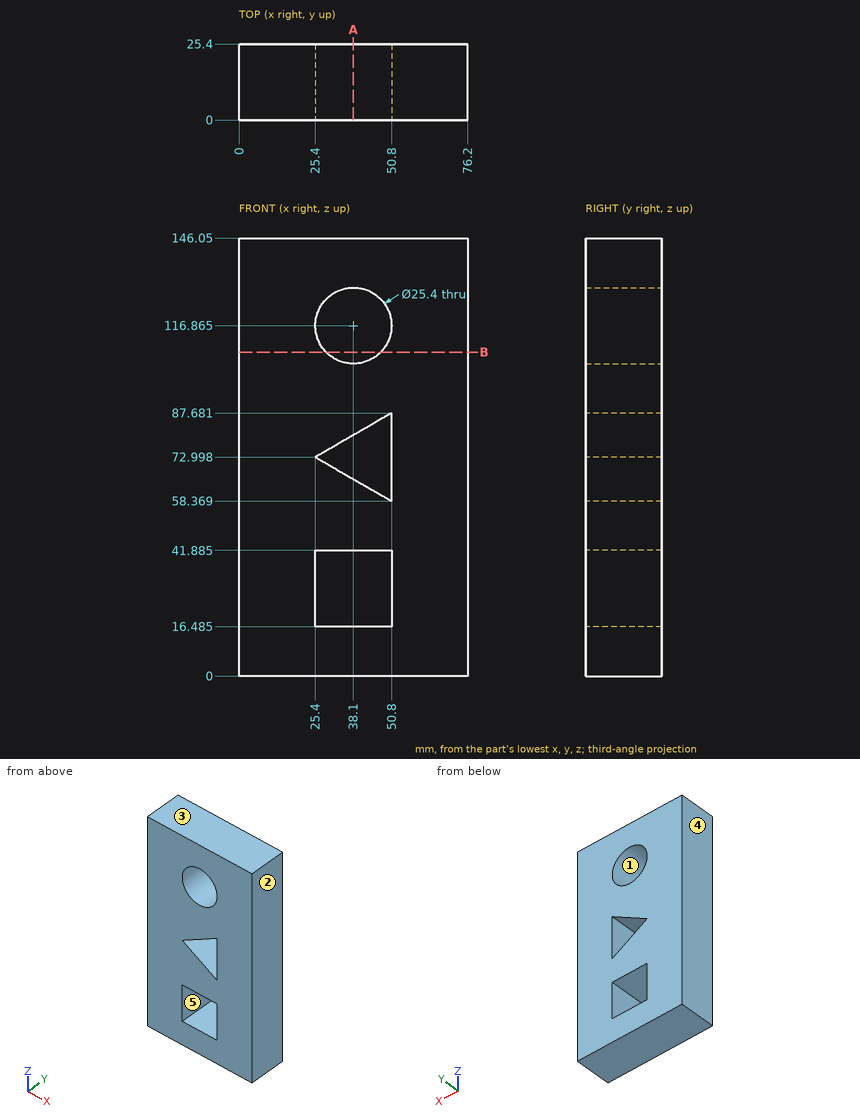
The drawing under review shows one solid part. Ordinate dimensions are in mm from its lowest x, y, z. A direction names the side the tool comes from. Round coordinates to 2 decimals unless told otherwise and drop trailing zeros. Order: outer loops, then holes, each group sorted by start corner. A loop starts at its lowest first (then second) coordinate and runs counter-clockwise, first axis right, second up. Notation, with made-up numbers: (56, -24) -> (84, -24) arc R21 cw to (84, 14) -> close; hole circle Ø1 at (-2, 20). An arc over 180 degrees is marked (long way). Use a Markdown table: item, result.
Q1. For line 1 (X direction, y = 7, z = 33); line 2 (X direction, y = 16.5, z = 86.5) (1 decimal), list the stretches that pass through material, from the lowest coordinate up.
Values:
| item | result |
|---|---|
| line 1 | x = 0 to 25.4, 50.8 to 76.2 |
| line 2 | x = 0 to 48.8, 50.8 to 76.2 |
Q2. We need section B-B on z = 108. Write out the cut boundary in (x, y).
Values:
| item | result |
|---|---|
| outline | (0, 0) -> (29.01, 0) -> (29.01, 25.4) -> (0, 25.4) -> close; (47.19, 0) -> (76.2, 0) -> (76.2, 25.4) -> (47.19, 25.4) -> close |
Q3. We need section A-A on x = 38.1. State how many separate pieces and enclosed holes the cut face has, then the cut area to 3 significant figures.
Values:
| item | result |
|---|---|
| separate pieces | 4 |
| enclosed holes | 0 |
| area | 2,050 mm^2 |
Q4. Tool access review of the marked faces 4 and 5: name each direction out of +Z, -Z, +X, -X, +Y, -Y from which nothing blocks a thin tool from reaching the whole face with its end or side.
Values:
| item | result |
|---|---|
| face 4 | +Z, -Z, -X, +Y, -Y |
| face 5 | +Y, -Y |
Q5. Mouldability with a two-part tool opening along X and no side actions: class the marked faces 1, 2 and 3 as +X half, -X half, draft (parallel to the pull), parting line (faces both ways), or undercut.
Values:
| item | result |
|---|---|
| face 1 | undercut |
| face 2 | +X half |
| face 3 | draft |
